```python
from build123d import *

# Parameters (mm, degrees)
F0_R     = 4.8
F0_R_2   = 2.5
F1_DEPTH = 6
F2_DEPTH = 40
F0_R_3   = 12.5
F3_DEPTH = 40
F4_DEPTH = 10
F0_R_4   = 13
F5_DEPTH = 11
F6_DEPTH = 10
F7_R     = 1


with BuildPart() as f1:
    # F0 (on Top) → F1 (new body)
    with BuildSketch(Plane.XY):
        Circle(F0_R)
        Circle(F0_R_2, mode=Mode.SUBTRACT)
    extrude(amount=-F1_DEPTH)

    # F0 (on Top) → F2 (join)
    with BuildSketch(Plane.XY):
        Polygon((2.640845, -11.350968), (10.521084, -5.012517), (10.478732, 5.100462), (2.545681, 11.372688), (-7.30432, 9.081049), (-11.654019, -0.048806), (-7.228004, -9.141909), align=None)
        Circle(F0_R, mode=Mode.SUBTRACT)
        Circle(F0_R)
        Circle(F0_R_2, mode=Mode.SUBTRACT)
    extrude(amount=F2_DEPTH)

    # F0 (on Top) → F3 (join)
    with BuildSketch(Plane.XY):
        Circle(F0_R_3)
        Polygon((10.478732, 5.100462), (10.521084, -5.012517), (2.640845, -11.350968), (-7.228004, -9.141909), (-11.654019, -0.048806), (-7.30432, 9.081049), (2.545681, 11.372688), align=None, mode=Mode.SUBTRACT)
    extrude(amount=F3_DEPTH)

    # F0 (on Top) → F4 (cut)
    with BuildSketch(Plane.XY):
        Circle(F0_R_3)
        Polygon((10.478732, 5.100462), (10.521084, -5.012517), (2.640845, -11.350968), (-7.228004, -9.141909), (-11.654019, -0.048806), (-7.30432, 9.081049), (2.545681, 11.372688), align=None, mode=Mode.SUBTRACT)
    extrude(amount=F4_DEPTH, mode=Mode.SUBTRACT)

    # F0 (on Top) → F5 (join)
    with BuildSketch(Plane.XY):
        Circle(F0_R_4)
        Circle(F0_R_3, mode=Mode.SUBTRACT)
    extrude(amount=F5_DEPTH)

    # F0 (on Top) → F6 (cut)
    with BuildSketch(Plane.XY):
        Circle(F0_R_4)
        Circle(F0_R_3, mode=Mode.SUBTRACT)
    extrude(amount=F6_DEPTH, mode=Mode.SUBTRACT)

    # F7
    f7_edges = [f1.edges().sort_by_distance(p)[0] for p in [
        (-4.8, 0, -6),
    ]]
    fillet(f7_edges, radius=F7_R)


solid = f1.part
```
Build history of the part. All positions in model axes, mm. A direction names the side the tool comes from. Give positions to 0.01 mm unless a question says otherwise; leave off trailing zeros. Loops run counter-clockwise (first coordinate to the right, second up) from the corner with the lowest first, then second, coordinate; pieces in that order, holes last.
Item 1: Slice it at D-D, the plane x = 6.75. List the corners of the cut face in (y, z).
Answers follow:
outline: (-11.11, 10) - (-8.05, 10) - (-8.05, 0) - (8.05, 0) - (8.05, 10) - (11.11, 10) - (11.11, 11) - (10.52, 11) - (10.52, 40) - (-10.52, 40) - (-10.52, 11) - (-11.11, 11) - close
Item 2: Drill centre lines: line 1 (Y direction, x = 0, z = 29); line 2 (Z direction, x = 5.75, y = 11); line 3 (X direction, y = 0.25, z = 32.5). Where is each one in solid material? Low to high.
Answers follow:
line 1: y = -12.5 to -2.5, 2.5 to 12.5
line 2: z = 10 to 40
line 3: x = -12.5 to -2.49, 2.49 to 12.5
Item 3: Slice it at A-A, the plane x = 0. List the corners of the cut face in (y, z).
Answers follow:
outline: (-13, 10) - (-10.76, 10) - (-10.76, 0) - (-4.8, 0) - (-4.8, -5) arc R1 ccw to (-3.8, -6) - (-2.5, -6) - (-2.5, 40) - (-12.5, 40) - (-12.5, 11) - (-13, 11) - close; (2.5, -6) - (3.8, -6) arc R1 ccw to (4.8, -5) - (4.8, 0) - (10.78, 0) - (10.78, 10) - (13, 10) - (13, 11) - (12.5, 11) - (12.5, 40) - (2.5, 40) - close
Item 4: Slice it at B-B, the plane z = 3. List the corners of the cut face in (x, y), and give its area (3 significant figures).
Answers follow:
outline: (-11.65, -0.05) - (-7.23, -9.14) - (2.64, -11.35) - (10.52, -5.01) - (10.48, 5.1) - (2.55, 11.37) - (-7.3, 9.08) - close; hole circle Ø5 at (0, 0)
area: 352 mm2
Item 5: Flat gauge pins, fed straight in: pin 1 (4 mm diameter, centred on y = -0.5, z = 14, fed in from +X); pin 2 (10 mm diameter, centred on y = -9, z = 35, fed in from +X); pin 3 (5 mm diameter, centred on x = -4.5, z = 17.5, fed in from -Y). Where does each tip first touch, or does it go through?
Answers follow:
pin 1: stops at x = 12.5
pin 2: stops at x = 11.84
pin 3: stops at y = -12.34
Item 6: Pull direction Y, two halves, no side cores. Call faces 5 (the face through (-10.316, -7.91, 10.493)), 6 (the face through (-0.54, -2.44, 16.68)), 7 (the face through (-2.45, 10.21, 4.93)): released by +Y, released by -Y, zero draft, split by the parting line, or undercut.
Answers follow:
face 5: split by the parting line
face 6: undercut
face 7: released by +Y
Item 7: Slice it at C-C, the plane y = 6.75. List the corners of the cut face in (x, z).
Answers follow:
outline: (-11.11, 10) - (-8.41, 10) - (-8.41, 0) - (8.39, 0) - (8.39, 10) - (11.11, 10) - (11.11, 11) - (10.52, 11) - (10.52, 40) - (-10.52, 40) - (-10.52, 11) - (-11.11, 11) - close
Item 8: Which spindle directions (+Z, -Z, +X, -X, +Y, -Y) get a long thin tool onto all of the face, cutting with end or side? Do faces 1 (the face through (6.636, -8.137, 4.93)), 2 (the face through (-9.51, 4.45, 4.93)), 3 (the face through (2.58, 4.05, -2.46)), 4 (the face through (11.923, 3.755, 25.297)). Say none if no direction does.
Answers follow:
face 1: -Z, +X, -Y
face 2: -Z, -X, +Y
face 3: -Z
face 4: +Z
